from build123d import *

# Parameters (mm, degrees)
EXTRUDE_1_DEPTH = 3


with BuildPart() as part:
    # 스케치1 → 보스-돌출1 (new body)
    with BuildSketch(Plane.XY):
        with BuildLine():
            Line((-1.455, 7.601440101), (1.455, 7.601440101))
            Line((1.455, 7.601440101), (1.455, 4.601440101))
            ThreePointArc((1.455, 4.601440101), (4.825998397, 0.003934023), (1.4625, -4.599061834))
            Line((1.4625, -4.599061834), (1.4625, -10.726759518))
            ThreePointArc((1.4625, -10.726759518), (0, 10.826), (-1.4625, -10.726759518))
            Line((-1.4625, -10.726759518), (-1.4625, -4.599061834))
            ThreePointArc((-1.4625, -4.599061834), (-4.825998397, 0.003934023), (-1.455, 4.601440101))
            Line((-1.455, 4.601440101), (-1.455, 7.601440101))
        make_face()
    extrude(amount=EXTRUDE_1_DEPTH)


solid = part.part
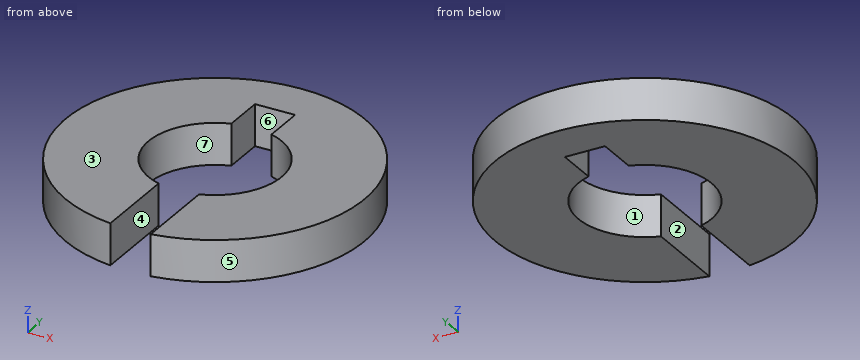
Here's how the part is built. I have some questions about the finished solid (model axes, mm). Face numbers are marked on the shaded views. A direction names the side the tool comes from. Coordinates: 2 decimals unless noted, no trailing zeros. Loops run counter-clockwise (first coordinate to the right, second up) from the corner with the lowest first, then second, coordinate; pieces in that order, holes last. Notation, with made-up numbers: (23.25, -17) -> (81.25, -17) arc R27 cw to (81.25, 6) -> close; hole circle Ø9 at (63, 60.5). An arc over 180 degrees is marked (long way). Use one line per item in the form item = value. Start each with the question number.
(1) On a 3-axis mill with a long thin cutter (end or side, diameter ignored), from which of +Z, -Z, +X, -X, +Y, -Y can I reach the whole of each face in a straight line? I mean the marked faces 1, 2 and 3. Say none if no direction works.
(2) If we section it at B-B (x = 3.75): Please give me the cut outline in (y, z), then the cut area to 3 significant figures.
(3) If we section it at A-A (y = 0): Please give me the cut outline in (x, z), then the cut area to 3 significant figures.
(4) If we section it at C-C (z = 1.1): Please give me the cut outline in (x, y) (1 decimal), then the cut area to 3 significant figures.
(5) We'd pull the mould along Y, two halves only. Please class the marked faces 4, 5, 6 and 7: pulls with the +Y half, pulls with the -Y half, needs draft (parallel to the pull), parting line crosses it, or undercut.
(6) If we section it at D-D (x = 0): Please give me the cut outline in (y, z).
(7) Please list where these lines run through material, in increasing order: line 1 along Y through (x, z) = (3, 2.05); line 2 along X through (y, z) = (-9.5, 1.05); line 3 along X through (y, z) = (7, 1.2) (3 decimals).
(8) Will this pin go through, and if not, where does the flat tip stop? pin 1 (0.9 mm diameter, centred on y = 7, z = 1.5, fed in from +X).
Verdict:
q1.face_1 = +Z, -Z
q1.face_2 = +Z, -Z, -Y
q1.face_3 = +Z, +X, -X, +Y, -Y
q2.outline = (-10.16, 0) -> (-3.04, 0) -> (-3.04, 3) -> (-10.16, 3) -> close; (3.04, 0) -> (10.16, 0) -> (10.16, 3) -> (3.04, 3) -> close
q2.area = 42.7 mm²
q3.outline = (-10.83, 0) -> (-4.83, 0) -> (-4.83, 3) -> (-10.83, 3) -> close; (4.83, 0) -> (10.83, 0) -> (10.83, 3) -> (4.83, 3) -> close
q3.area = 36.0 mm²
q4.outline = (-1.5, -10.7) -> (-1.5, -4.6) arc R4.8 cw to (-1.5, 4.6) -> (-1.5, 7.6) -> (1.5, 7.6) -> (1.5, 4.6) arc R4.8 cw to (1.5, -4.6) -> (1.5, -10.7) arc R10.8 ccw (long way) to start
q4.area = 269 mm²
q5.face_4 = needs draft
q5.face_5 = parting line crosses it
q5.face_6 = pulls with the -Y half
q5.face_7 = undercut
q6.outline = (7.6, 0) -> (10.83, 0) -> (10.83, 3) -> (7.6, 3) -> close
q7.line_1 = -10.4 to -3.78, 3.78 to 10.4
q7.line_2 = -5.19 to -1.46, 1.46 to 5.19
q7.line_3 = -8.258 to -1.455, 1.455 to 8.258
q8.pin_1 = 8.62
